```python
from build123d import *

# Parameters (mm, degrees)
F0_W     = 28
F0_H     = 8
F1_DEPTH = 0.25
F2_SIZE  = 0.5
F3_R     = 1.8
F4_DEPTH = 0.251


with BuildPart() as f1:
    # F0 (on Top) → F1 (new body)
    with BuildSketch(Plane.XY):
        Rectangle(F0_W, F0_H)
    extrude(amount=F1_DEPTH)

    # F2
    f2_edges = [f1.edges().sort_by_distance(p)[0] for p in [
        (-14, -4, 0.125),
        (-14, 4, 0.125),
        (14, -4, 0.125),
        (14, 4, 0.125),
    ]]
    chamfer(f2_edges, length=F2_SIZE)

    # F3 (on face) → F4 (cut, through all)
    with BuildSketch(Plane.XY.offset(0.25)):
        with Locations((-9.45, 0)):
            Circle(F3_R)
        with Locations((9.45, 0)):
            Circle(F3_R)
    extrude(amount=-F4_DEPTH, mode=Mode.SUBTRACT)


solid = f1.part
```
Build history of the part. All positions in model axes, mm. Coordinates: 2 decimals unless noted, no trailing zeros. Order: outer loops, then holes, each group sorted by start corner. A loop starts at its lowest first (then second) coordinate and runs counter-clockwise, first axis right, second up. Notation, with made-up numbers: M 24,70 L 41,70 A8 cw 41,77 Z; hole C -14.75,47 d5. An arc over 180 degrees is marked long. One line per question, with ' | ' between items. Start each with the question number.
1. Cut at A-A (z = 0.15). Write the cut outline in (x, y), plus the area to 3 significant figures.
2. Cut at D-D (y = 1.25). Write the cut outline in (x, z).
3. Flat gauge pin, fed straight in: P1, Ø1.5, axis at x = 9, y = 0, coming from the -Z side. Where does the tip first touch, or does it go through?
4. Cut at B-B (y = 0). Write the cut outline in (x, z).
5. Cut at C-C (x = -9.45). Write the cut outline in (y, z), plus the area to 3 significant figures.
6. Wall check: line 1 along X through (y, z) = (-0.25, 0.1); line 2 along X through (y, z) = (1.5, 0.15); line 3 along Y through (x, z) = (-9.45, 0.2). Give the ranges that are in metal, low to high. Write a range as [from, to].
The answers:
1) outline: M -14,-3.5 L -13.5,-4 L 13.5,-4 L 14,-3.5 L 14,3.5 L 13.5,4 L -13.5,4 L -14,3.5 Z; hole C -9.45,0 d3.6; hole C 9.45,0 d3.6 | area: 203 mm2
2) outline: M -14,0 L -10.75,0 L -10.75,0.25 L -14,0.25 Z; M -8.15,0 L 8.15,0 L 8.15,0.25 L -8.15,0.25 Z; M 10.75,0 L 14,0 L 14,0.25 L 10.75,0.25 Z
3) P1: passes through
4) outline: M -14,0 L -11.25,0 L -11.25,0.25 L -14,0.25 Z; M -7.65,0 L 7.65,0 L 7.65,0.25 L -7.65,0.25 Z; M 11.25,0 L 14,0 L 14,0.25 L 11.25,0.25 Z
5) outline: M -4,0 L -1.8,0 L -1.8,0.25 L -4,0.25 Z; M 1.8,0 L 4,0 L 4,0.25 L 1.8,0.25 Z | area: 1.10 mm2
6) line 1: x = [-14, -11.23], [-7.67, 7.67], [11.23, 14] | line 2: x = [-14, -10.44], [-8.46, 8.46], [10.44, 14] | line 3: y = [-4, -1.8], [1.8, 4]
